CAD build for the part. Positions are in the model's coordinates, mm. Face numbers are marked on the shaded views. Round coordinates to 2 decimals unless told otherwise and drop trailing zeros. Loops run counter-clockwise (first coordinate to the right, second up) from the corner with the lowest first, then second, coordinate; pieces in that order, holes last. Notation, with made-up numbers: M -39,67 L -31,67 A18 cw -31,83 Z; hole C 71,-24.75 d4. An arc over 180 degrees is marked long. Put each result on its own line as item: value. Start each with the question number.
from build123d import *

# Parameters (mm, degrees)
SKETCH1_R           = 26.75
BOSS_EXTRUDE1_DEPTH = 10
SKETCH2_R           = 24.25
CUT_EXTRUDE3_DEPTH  = 5
CUT_EXTRUDE5_DEPTH  = 6
SKETCH8_W           = 12
SKETCH8_H           = 20
BOSS_EXTRUDE2_DEPTH = 4
SKETCH9_R           = 1.65
CUT_EXTRUDE6_DEPTH  = 15
SKETCH9_3_R         = 1.65
CUT_EXTRUDE7_DEPTH  = 15


with BuildPart() as part:
    # Sketch1 → Boss-Extrude1 (new body)
    with BuildSketch(Plane(origin=(0, 0, 0), x_dir=(1, 0, 0), z_dir=(0, 1, 0))):
        with Locations(Location((0, 0, 0), (0, 0, 270))):
            Circle(SKETCH1_R)
    extrude(amount=BOSS_EXTRUDE1_DEPTH)

    # Sketch2 → Cut-Extrude3 (cut)
    with BuildSketch(Plane(origin=(0, 10, 0), x_dir=(1, 0, 0), z_dir=(0, 1, 0))):
        with Locations(Location((0, 0, 0), (0, 0, 270))):
            Circle(SKETCH2_R)
    extrude(amount=-CUT_EXTRUDE3_DEPTH, mode=Mode.SUBTRACT)

    # Sketch3 → Cut-Extrude5 (cut)
    with BuildSketch(Plane(origin=(0, 5, 0), x_dir=(1, 0, 0), z_dir=(0, 1, 0))):
        with BuildLine():
            Line((3.5, 3.039080618), (3.5, -3.039080618))
            ThreePointArc((3.5, -3.039080618), (0, -6.539080618), (-3.5, -3.039080618))
            Line((-3.5, -3.039080618), (-3.5, 3.039080618))
            ThreePointArc((-3.5, 3.039080618), (0, 6.539080618), (3.5, 3.039080618))
        make_face()
    extrude(amount=-CUT_EXTRUDE5_DEPTH, mode=Mode.SUBTRACT)

    # Sketch8 → Boss-Extrude2 (add)
    with BuildSketch(Plane.XZ):
        Rectangle(SKETCH8_W, SKETCH8_H)
    extrude(amount=BOSS_EXTRUDE2_DEPTH)

    # Sketch9 → Cut-Extrude6 (cut)
    with BuildSketch(Plane(origin=(0, 0, 0), x_dir=(1, 0, 0), z_dir=(0, 1, 0))):
        with Locations(Location((0, 3, 0), (0, 0, 270))):
            Circle(SKETCH9_R)
    extrude(amount=-CUT_EXTRUDE6_DEPTH, mode=Mode.SUBTRACT)

    # Sketch9_3 → Cut-Extrude7 (cut)
    with BuildSketch(Plane(origin=(0, 0, 0), x_dir=(1, 0, 0), z_dir=(0, 1, 0))):
        with Locations(Location((0, 3, 0), (0, 0, 270))):
            Circle(SKETCH9_3_R)
        with Locations(Location((0, -3, 0), (0, 0, 270))):
            Circle(SKETCH9_3_R)
    extrude(amount=-CUT_EXTRUDE7_DEPTH, mode=Mode.SUBTRACT)


solid = part.part
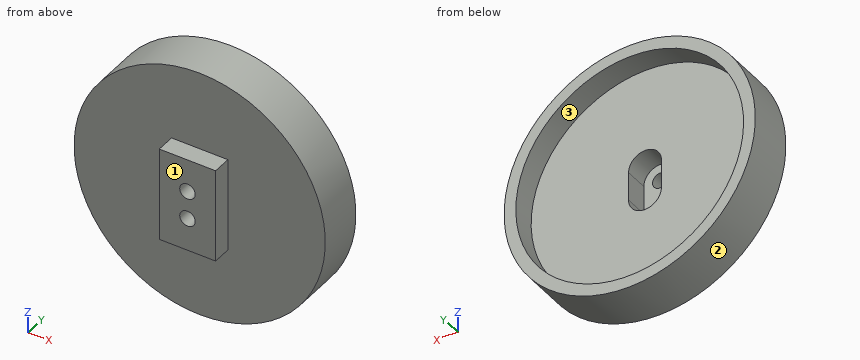
(1) Drill centre lines: line 1 along X through (y, z) = (6.45, 0); line 2 along X through (y, z) = (-1.25, 3); line 3 along Y through (x, z) = (2, -8). Where is each one in solid material? Low to high.
(2) Flat gauge pins, fed straight in: pin 1 Ø1.2 at (x, y) = (1.5, -1.5) entering from -Z; pin 2 Ø4.5 at (y, z) = (-2.5, 1.5) entering from -X; pin 3 Ø24 at (x, z) = (1, 4.5) entering from +Y; pin 4 Ø4 at (x, z) = (0, 3) entering from -Y. Where does each tip first touch, or does it go through?
(3) Cut at A-A on x = 0. List the corners of the cut face in (y, z).
(4) Cut at D-D on x = -14. List the corners of the cut face in (y, z).
(5) Cut at C-C on z = 0. List the corners of the cut face in (x, y).
(6) Cut at B-B on y = 8.75. List the corners of the cut face in (x, z), and give its area (3 significant figures).
(7) Mould opens along X. For the marked faces 1, 2 and 3 say: +X half, -X half, draft (parallel to the pull), parting line (faces both ways), or undercut.
Taken from the geometry:
1. line 1: -26.75 to -24.25, 24.25 to 26.75
1. line 2: -6 to -1.65, 1.65 to 6
1. line 3: -4 to 5
2. pin 1: z = -10
2. pin 2: x = -6
2. pin 3: y = 5
2. pin 4: y = -4
3. outline: M -4,-10 L 0,-10 L 0,-26.75 L 10,-26.75 L 10,-24.25 L 5,-24.25 L 5,-6.54 L 0,-6.54 L 0,-4.65 L -4,-4.65 Z; M -4,-1.35 L 0,-1.35 L 0,1.35 L -4,1.35 Z; M -4,4.65 L 0,4.65 L 0,6.54 L 5,6.54 L 5,24.25 L 10,24.25 L 10,26.75 L 0,26.75 L 0,10 L -4,10 Z
4. outline: M 0,-22.79 L 10,-22.79 L 10,-19.8 L 5,-19.8 L 5,19.8 L 10,19.8 L 10,22.79 L 0,22.79 Z
5. outline: M -26.75,0 L -6,0 L -6,-4 L 6,-4 L 6,0 L 26.75,0 L 26.75,10 L 24.25,10 L 24.25,5 L 3.5,5 L 3.5,0 L -3.5,0 L -3.5,5 L -24.25,5 L -24.25,10 L -26.75,10 Z
6. outline: C 0,0 d53.5; hole C 0,0 d48.5
6. area: 401 mm2
7. face 1: draft
7. face 2: parting line
7. face 3: undercut
